Read the model definition and answer for the solid it produces. Units are mm, in the model's axes. A direction names the side the tool comes from. Coordinates: 2 decimals unless noted, no trailing zeros. Write each loop counter-clockwise with the first axis right and the second up, starting at its lowest first coordinate (ties: lowest second). Pieces come first, ordered by that corner, then holes.
(1) Section A-A on x = 33.25 is taken. Write down the section's boundary in (y, z), then the cut area to 3 significant figures.
(2) Which of the six approach directions +Z, -Z, +X, -X, +Y, -Y give full straight-line access (tool end or side, diameter ignored) to faces 4 (the flat face through (337.3, 116, 3)), 5 (the flat face through (19.25, 90, 3)), 6 (the flat face through (169, 67, 6.35))?
(3) Section B-B on y = 90.1 is taken. Write down the section's boundary in (x, z).
(4) Section D-D on y = 23.2 is taken. Write down the section's boundary in (x, z).
(5) Section C-C on z = 3.5 is taken. State how many separate pieces and enclosed holes the cut face has, then the cut area to 3 significant figures.
(6) The mould has two halves that part along X. Classify faces 1 (the flat face through (342, 52, 3)), 2 (the flat face through (67, 70.2, 3)), 3 (the flat face through (169, 0, 3)): +X half, -X half, draft (parallel to the pull), parting line (faces both ways), or undercut.
(7) Find the intervals of material crossed by probe 1 along Y at (x, z) = (33.25, 5.25); probe 2 along Y at (x, z) = (169.75, 3); probe 3 along X at (y, z) = (76.5, 2), in increasing order.
(8) Given pin 1 (3 mm diameter, centred on y = 111, z = 2.5, fed in from +X), flat-ended and moving along its own axis, determine where the tip first touches the part or whether it passes through.
from build123d import *

# Parameters (mm, degrees)
SKETCH1_R           = 1.9
SKETCH1_R_2         = 8
SKETCH1_R_3         = 4.55
SKETCH1_W           = 97.5
SKETCH1_H           = 39.8
BOSS_EXTRUDE1_DEPTH = 6.35


with BuildPart() as part:
    # Sketch1 → Boss-Extrude1 (new body)
    with BuildSketch(Plane.XY):
        Polygon((0, 0), (342, 0), (342, 105), (337.3, 105), (337.3, 127.3), (315, 127.3), (315, 132), (0, 132), align=None)
        with Locations((114.499995121, 117.600002885)):
            Circle(SKETCH1_R, mode=Mode.SUBTRACT)
        with Locations((114.499995121, 62.6)):
            Circle(SKETCH1_R, mode=Mode.SUBTRACT)
        with Locations((21.499995121, 62.6)):
            Circle(SKETCH1_R, mode=Mode.SUBTRACT)
        with Locations((21.499995121, 117.600002885)):
            Circle(SKETCH1_R, mode=Mode.SUBTRACT)
        with Locations((146.75, 90.1)):
            Circle(SKETCH1_R_2, mode=Mode.SUBTRACT)
        with Locations((169.75, 90.1)):
            Circle(SKETCH1_R_2, mode=Mode.SUBTRACT)
        with Locations((33.25, 23.2)):
            Circle(SKETCH1_R_3, mode=Mode.SUBTRACT)
        with Locations((68, 90.1)):
            Rectangle(SKETCH1_W, SKETCH1_H, mode=Mode.SUBTRACT)
    extrude(amount=BOSS_EXTRUDE1_DEPTH)


solid = part.part
Response:
1. outline: (0, 0) - (18.65, 0) - (18.65, 6.35) - (0, 6.35) - close; (27.75, 0) - (70.2, 0) - (70.2, 6.35) - (27.75, 6.35) - close; (110, 0) - (132, 0) - (132, 6.35) - (110, 6.35) - close
1. area: 528 mm2
2. face 4: +Z, -Z, +X, +Y
2. face 5: +Z, -Z
2. face 6: +Z, +X, -X, +Y, -Y
3. outline: (0, 0) - (19.25, 0) - (19.25, 6.35) - (0, 6.35) - close; (116.75, 0) - (138.75, 0) - (138.75, 6.35) - (116.75, 6.35) - close; (154.75, 0) - (161.75, 0) - (161.75, 6.35) - (154.75, 6.35) - close; (177.75, 0) - (342, 0) - (342, 6.35) - (177.75, 6.35) - close
4. outline: (0, 0) - (28.7, 0) - (28.7, 6.35) - (0, 6.35) - close; (37.8, 0) - (342, 0) - (342, 6.35) - (37.8, 6.35) - close
5. separate pieces: 1
5. enclosed holes: 8
5. area: 40,500 mm2
6. face 1: +X half
6. face 2: undercut
6. face 3: draft
7. probe 1: y = 0 to 18.65, 27.75 to 70.2, 110 to 132
7. probe 2: y = 0 to 82.1, 98.1 to 132
7. probe 3: x = 0 to 19.25, 116.75 to 342
8. pin 1: stops at x = 337.3
